Model file for the job. Use its own axes, mm. Coordinates: 2 decimals unless noted, no trailing zeros. Order: outer loops, then holes, each group sorted by start corner. A loop starts at its lowest first (then second) coordinate and runs counter-clockwise, first axis right, second up. Notation, with made-up numbers: (76, 76) -> (103, 76) arc R8 cw to (103, 81) -> close; hole circle Ø7 at (38.5, -2.75). An arc over 180 degrees is marked (long way). Use CSV: the item, a comma, the result in double quotes. Start each with the question number.
(1) Cut at A-A on y = 0.95. Write the cut outline in (x, z).
(2) Cut at B-B on x = 285.5. Write the cut outline in (y, z).
(3) Probe L1, parallel to X at y = 1.3, z = 181.5. List the from-to ranges inside material, lowest first.
(4) Pin check, flat tips, straight feed: pin 1 Ø0.6 at (y, z) = (1, -186) entering from +X; pin 2 Ø0.6 at (x, y) = (290, 1.5) entering from -Z; pin 3 Ø1 at (x, y) = (298, 1.5) entering from +Z. Stop position of each tip, or through.
(5) Cut at C-C on z = 167. Write the cut outline in (x, y).
```python
from build123d import *

# Parameters (mm, degrees)
BOSS_EXTRUDE1_DEPTH = 2


with BuildPart() as part:
    # Sketch1 → Boss-Extrude1 (new body)
    with BuildSketch(Plane(origin=(0, 0, 0), x_dir=(1, 0, 0), z_dir=(0, 1, 0))):
        Polygon((-325.499342603, 150.901111002), (-307.000657397, 150.901111002), (-305.400657397, 150.901111002), (-305.400657397, 179.901111002), (-276.400657397, 179.901111002), (-276.400657397, 199.998908398), (276.400657397, 199.998908398), (276.400657397, 179.901111002), (305.400657397, 179.901111002), (305.400657397, 150.901111002), (325.499342603, 150.901111002), (325.499342603, -150.901091602), (305.400657397, -150.901091602), (305.400657397, -179.901091602), (276.400657397, -179.901091602), (276.400657397, -199.998908398), (-276.400657397, -199.998908398), (-276.400657397, -179.901091602), (-305.400657397, -179.901091602), (-305.400657397, -150.901091602), (-325.499342603, -150.901091602), align=None)
    extrude(amount=BOSS_EXTRUDE1_DEPTH)


solid = part.part
```
Outcome:
1,outline,"(-325.5, -150.9) -> (-305.4, -150.9) -> (-305.4, -179.9) -> (-276.4, -179.9) -> (-276.4, -200) -> (276.4, -200) -> (276.4, -179.9) -> (305.4, -179.9) -> (305.4, -150.9) -> (325.5, -150.9) -> (325.5, 150.9) -> (305.4, 150.9) -> (305.4, 179.9) -> (276.4, 179.9) -> (276.4, 200) -> (-276.4, 200) -> (-276.4, 179.9) -> (-305.4, 179.9) -> (-305.4, 150.9) -> (-325.5, 150.9) -> close"
2,outline,"(0, -179.9) -> (2, -179.9) -> (2, 179.9) -> (0, 179.9) -> close"
3,L1,"-276.4 to 276.4"
4,pin 1,"x = 276.4"
4,pin 2,"z = -179.9"
4,pin 3,"z = 179.9"
5,outline,"(-305.4, 0) -> (305.4, 0) -> (305.4, 2) -> (-305.4, 2) -> close"
